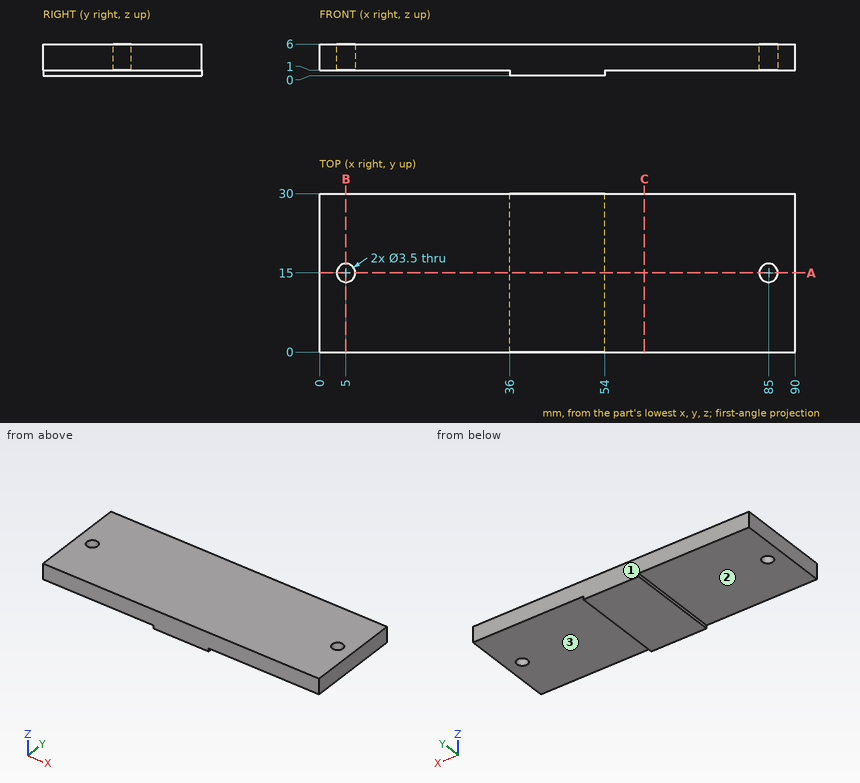
Print and shaded views of the part. All mm, measured from the part's lowest x, y and z. A direction names the side the tool comes from. Coordinates: 2 decimals unless noted, no trailing zeros. Order: outer loops, then holes, each group sorted by start corner. A loop starts at its lowest first (then second) coordinate and runs counter-clockwise, first axis right, second up. Notation, with made-up numbers: M 6,39.25 L 27,39.25 A13 ccw 27,46.25 Z; hole C -3.75,55.25 d11. An arc over 180 degrees is marked long. Write each question's results on one line, items separated by ' | '. Start each with the question number.
Q1. Which spindle directions (+Z, -Z, +X, -X, +Y, -Y) get a long thin tool onto all of the face, cutting with end or side? Do the marked faces 1, 2 and 3. Say none if no direction does.
Q2. Cut at B-B (x = 5). List the corners of the cut face in (y, z), then the cut area to 4 significant figures.
Q3. Cut at A-A (y = 15). List the corners of the cut face in (x, z).
Q4. Cut at C-C (x = 61.5). List the corners of the cut face in (y, z).
Q5. Drill centre lines: probe 1 along Y at (x, z) = (85, 4.3); probe 2 along Z at (x, y) = (62, 27); probe 3 along X at (y, z) = (26, 0.55). Where is each one in solid material? Low to high. Write a range as from..to.
Q6. Flat gauge pins, fed straight in: P1, Ø4, axis at x = 5, y = 15, coming from the -Z side; P2, Ø3, axis at x = 85, y = 15, coming from the +Z side. Where does each tip first touch, or does it go through?
Found:
1) face 1: +Z, -Z, +X, -X, +Y | face 2: -Z, -X, +Y, -Y | face 3: -Z, +X, +Y, -Y
2) outline: M 0,1 L 13.25,1 L 13.25,6 L 0,6 Z; M 16.75,1 L 30,1 L 30,6 L 16.75,6 Z | area: 132.5 mm²
3) outline: M 0,1 L 3.25,1 L 3.25,6 L 0,6 Z; M 6.75,1 L 36,1 L 36,0 L 54,0 L 54,1 L 83.25,1 L 83.25,6 L 6.75,6 Z; M 86.75,1 L 90,1 L 90,6 L 86.75,6 Z
4) outline: M 0,1 L 30,1 L 30,6 L 0,6 Z
5) probe 1: 0..13.25, 16.75..30 | probe 2: 1..6 | probe 3: 36..54
6) P1: z = 1 | P2: through
